Part print with two shaded views. Sizes in mm from the minimum x, y, z corner. A direction names the side the tool comes from. Round coordinates to 2 decimals unless told otherwise and drop trailing zeros. Loops run counter-clockwise (first coordinate to the right, second up) from the corner with the lowest first, then second, coordinate; pieces in that order, holes last. Notation, with made-up numbers: (85, 63) - (107, 63) arc R13 ccw to (107, 73) - close; hole circle Ø11 at (-33, 2). An arc over 180 degrees is marked (long way). Write each question's results on one line, items separated by ' | '. Start each with the question number.
(1) Cut at C-C, the plane z = 450.5. List the corners of the cut face in (x, y) (1 decimal).
(2) Cut at A-A, the plane x = 37. List the corners of the cut face in (y, z), then the cut area to 3 significant figures.
(3) Drill centre lines: L1, parallel to Z at x = 43, y = 116.5; L2, parallel to X at y = 66.5, z = 136.5; L3, parallel to Y at x = 5.5, z = 44. Where is each one in solid material? Low to high.
(4) Cut at D-D, the plane y = 255. List the corners of the cut face in (x, z), then the cut area to 3 significant figures.
(5) Cut at B-B, the plane y = 90. List the corners of the cut face in (x, z), then the cut area to 3 significant figures.
(6) Flat gauge pins, fed straight in: P1, Ø25, axis at x = 52, y = 229.5, coming from the +Z side; P2, Ø6, axis at y = 61, z = 372.5, coming from the -X side; P3, Ø6, axis at y = 76.5, z = 614.5, coming from the +X side; P4, Ø2, axis at x = 7.5, z = 430, coming from the +Y side. Where does each tip first touch, or does it go through?
(7) Tool access for the marked faces 1, 2 and 3: list every direction of +Z, -Z, +X, -X, +Y, -Y with a clear straight run to the whole face (end or side of a thin tool).
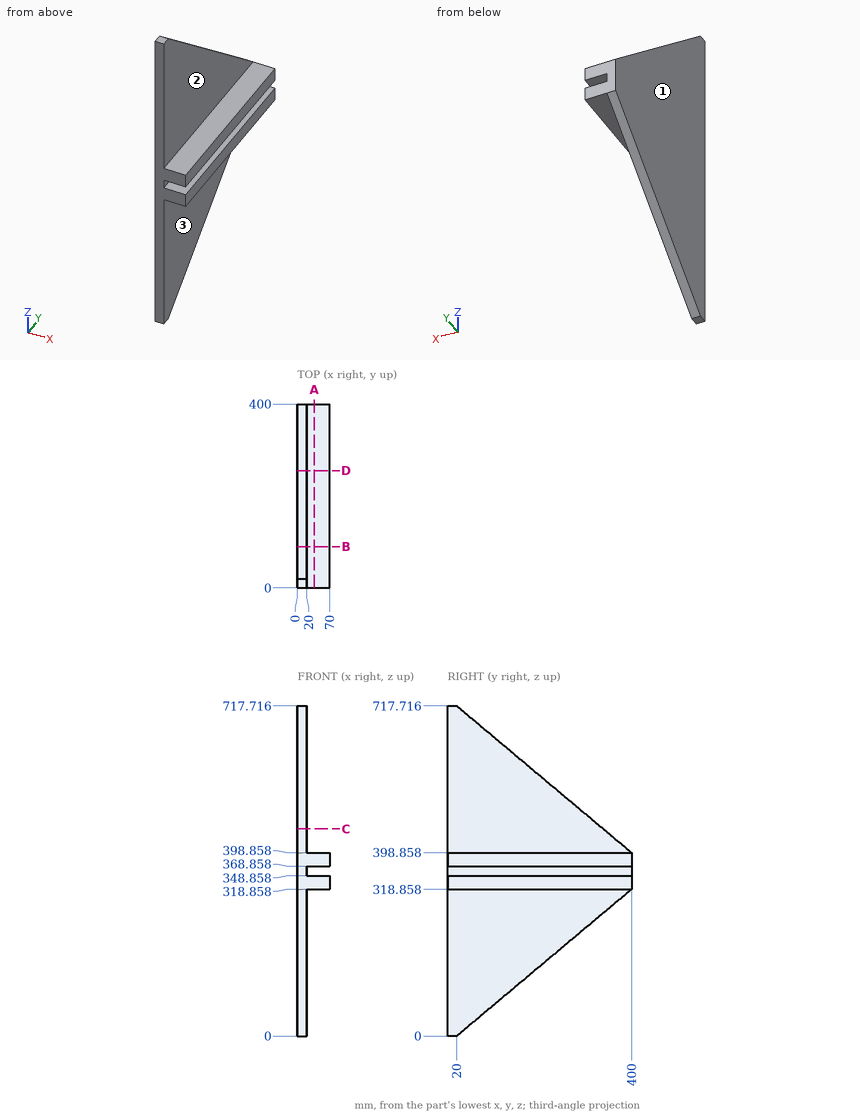
A:
1) outline: (0, 0) - (20, 0) - (20, 338.5) - (0, 338.5) - close
2) outline: (0, 318.86) - (400, 318.86) - (400, 348.86) - (0, 348.86) - close; (0, 368.86) - (400, 368.86) - (400, 398.86) - (0, 398.86) - close | area: 24,000 mm2
3) L1: 318.86 to 348.86, 368.86 to 398.86 | L2: 0 to 20 | L3: 0 to 72.44
4) outline: (0, 197.19) - (20, 197.19) - (20, 318.86) - (70, 318.86) - (70, 348.86) - (20, 348.86) - (20, 368.86) - (70, 368.86) - (70, 398.86) - (20, 398.86) - (20, 520.53) - (0, 520.53) - close | area: 9,470 mm2
5) outline: (0, 58.74) - (20, 58.74) - (20, 318.86) - (70, 318.86) - (70, 348.86) - (20, 348.86) - (20, 368.86) - (70, 368.86) - (70, 398.86) - (20, 398.86) - (20, 658.98) - (0, 658.98) - close | area: 15,000 mm2
6) P1: z = 398.86 | P2: x = 0 | P3: x = 20 | P4: y = 364.08
7) face 1: +Z, -Z, -X, +Y, -Y | face 2: +Z, +X, +Y, -Y | face 3: -Z, +X, +Y, -Y
